The model under review builds one solid part; all positions refer to its coordinate system, in mm. A direction names the side the tool comes from. Coordinates: 2 decimals unless noted, no trailing zeros. Order: outer loops, then holes, each group sorted by start corner. A loop starts at its lowest first (then second) coordinate and runs counter-clockwise, first axis right, second up. Notation, with made-up numbers: M 72,44.25 L 83,44.25 A8 cw 83,57.25 Z; hole C -27.75,80.25 d3. An arc over 180 degrees is marked long. Answer in a Markdown table with one row per item.
Autodesk Inventor part; units mm, degrees
ref_plane "YZ Plane" through (0, 0, 0) normal (1, 0, 0) x (0, 1, 0)
ref_plane "XZ Plane" through (0, 0, 0) normal (0, 1, 0) x (-1, 0, 0)
ref_plane "XY Plane" through (0, 0, 0) normal (0, 0, 1) x (1, 0, 0)
sketch "Sketch1" plane through (0, 0, 0) normal (0, 1, 0) x (-1, 0, 0)
  line L0 (0, 0) -> (47.635, 0)
  line L1 (47.635, 0) -> (47.635, -52.715)
  line L2 (47.635, -52.715) -> (0, -52.715)
  line L3 (0, -52.715) -> (0, 0)
  circle A0 centre (45.725, -1.91) radius 2.1
  circle A1 centre (45.725, -50.805) radius 2.1
  circle A2 centre (1.91, -1.91) radius 2.1
  circle A3 centre (1.91, -50.805) radius 2.1
  line L4 (47.635, 0) -> (51.445, 0)
  line L5 (51.445, 0) -> (51.445, -52.715)
  line L6 (51.445, -52.715) -> (47.635, -52.715)
  line L7 (47.635, -52.715) -> (47.635, 0)
  line L8 (0, 0) -> (-3.81, 0)
  line L9 (-3.81, 0) -> (-3.81, -56.525)
  line L10 (-3.81, -56.525) -> (0, -56.525)
  line L11 (0, -56.525) -> (0, 0)
  line L12 (51.445, -52.715) -> (-6.35, -52.715)
  line L13 (-6.35, -52.715) -> (-6.35, -56.525)
  line L14 (-6.35, -56.525) -> (51.445, -56.525)
  line L15 (51.445, -56.525) -> (51.445, -52.715)
  line L16 (-3.81, 0) -> (51.445, 0)
  line L17 (51.445, 0) -> (51.445, 3.81)
  line L18 (51.445, 3.81) -> (-3.81, 3.81)
  line L19 (-3.81, 3.81) -> (-3.81, 0)
  point P0 (0, -52.715)
  point P1 (0, -51.6779)
  point P2 (0, -49.9321)
  point P3 (0, -2.7829)
  point P4 (0, -1.0371)
  point P5 (-3.81, -77.675)
  point P6 (-3.81, -52.715)
  point P7 (0, -52.715)
  point P8 (1.0371, -52.715)
  point P9 (2.7829, -52.715)
  point P10 (0, -52.715)
  point P11 (0, -56.525)
  point P12 (0, -56.525)
  dimension "d0" = 52.715
  dimension "d1" = 47.635
  dimension "d3" = 4.2
  dimension "d4" = 4.2
  dimension "d6" = 1.91
  dimension "d7" = 1.91
  dimension "d8" = 1.91
  dimension "d9" = 4.2
  dimension "d10" = 4.2
  dimension "d11" = 1.91
  dimension "d12" = 1.91
  dimension "d13" = 1.91
  dimension "d14" = 1.91
  dimension "d15" = 1.91
  dimension "d18" = 3.81
  dimension "d19" = 3.81
  dimension "d20" = 3.81
  dimension "d21" = 3.81
  dimension "d38" = 0
  dimension "d39" = 0
extrude "Extrusion5" add sketch "Sketch1" along normal blind 15 contours L8 L19 L18 L17 L4 L0 A0 A2 | L0 A2 L3 | L3 A2 A3 L12 L9 L8 | L0 A0 L1 A1 L2 A3 L3 A2 | L12 L11 L10 L9 | L3 A3 L2 | L2 A3 A1 L6 L15 L14 L11 | L0 L1 A0 | A0 L1 L4 L5 L6 A1 | L1 L2 A1 picked at (0.2904, -0.2904) picked at (0.2904, -52.4246) picked at (47.3446, -0.2904) picked at (47.3446, -52.4246)
sketch "Sketch6" plane through (0, 15, 0) normal (0, 1, 0) x (1, 0, 0)
  line L0 (-51.445, -3.81) -> (3.81, -3.81)
  line L1 (-51.445, -3.81) -> (-38.745, -3.81)
  line L2 (-38.745, -3.81) -> (-38.745, 8.89)
  line L3 (-38.745, 8.89) -> (-51.445, 8.89)
  line L4 (-51.445, 8.89) -> (-51.445, -3.81)
  line L5 (3.81, 56.525) -> (-51.445, 56.525)
  line L6 (-51.445, 56.525) -> (-38.745, 56.525)
  line L7 (-38.745, 56.525) -> (-38.745, 43.825)
  line L8 (-38.745, 43.825) -> (-51.445, 43.825)
  line L9 (-51.445, 43.825) -> (-51.445, 56.525)
  line L10 (3.81, -3.81) -> (3.81, 56.525)
  line L11 (3.81, 56.525) -> (-8.89, 56.525)
  line L12 (-8.89, 56.525) -> (-8.89, 43.825)
  line L13 (-8.89, 43.825) -> (3.81, 43.825)
  line L14 (3.81, 43.825) -> (3.81, 56.525)
  line L15 (3.81, -3.81) -> (-8.89, -3.81)
  line L16 (-8.89, -3.81) -> (-8.89, 8.89)
  line L17 (-8.89, 8.89) -> (3.81, 8.89)
  line L18 (3.81, 8.89) -> (3.81, -3.81)
  line L19 (3.81, 56.525) -> (-51.445, 56.525)
  line L20 (-51.445, 56.525) -> (-51.445, -3.81)
  line L21 (-51.445, -3.81) -> (3.81, -3.81)
  line L22 (3.81, -3.81) -> (3.81, 56.525)
  circle A0 centre (-1.91, 1.91) radius 2.1
  circle A1 centre (-45.725, 1.91) radius 2.1
  circle A2 centre (-45.725, 50.805) radius 2.1
  circle A3 centre (-1.91, 50.805) radius 2.1
  point P0 (0, 0)
  point P1 (3.81, 8.89)
  dimension "d42" = 12.7
  dimension "d43" = 12.7
  dimension "d44" = 12.7
  dimension "d45" = 12.7
  dimension "d46" = 12.7
  dimension "d47" = 12.7
extrude "Extrusion6" cut sketch "Sketch6" against normal blind 10 contours L2 L3 L20 L8 L7 L5 L12 L13 L10 L17 L16 L0
sketch "Sketch7" plane through (0, 0, 0) normal (0, -1, 0) x (1, 0, 0)
  line L0 (3.81, -56.525) -> (-51.445, -56.525)
  line L1 (3.81, 3.81) -> (3.81, -56.525)
  line L2 (-51.445, 3.81) -> (3.81, 3.81)
  line L3 (-51.445, -56.525) -> (-51.445, 3.81)
  circle A0 centre (-1.91, -1.91) radius 2.1
  circle A1 centre (-45.725, -1.91) radius 2.1
  circle A2 centre (-45.725, -50.805) radius 2.1
  circle A3 centre (-1.91, -50.805) radius 2.1
  line L4 (-8.89, 3.81) -> (3.81, 3.81)
  line L5 (3.81, 3.81) -> (-51.445, 3.81)
  line L6 (-51.445, 3.81) -> (-51.445, 6.35)
  line L7 (-51.445, 6.35) -> (3.81, 6.35)
  line L8 (3.81, 6.35) -> (3.81, 3.81)
  line L9 (-51.445, 6.35) -> (-53.985, 6.35)
  line L10 (-53.985, 6.35) -> (-53.985, -56.525)
  line L11 (-53.985, -56.525) -> (-51.445, -56.525)
  line L12 (-51.445, -56.525) -> (-51.445, 6.35)
  line L13 (-53.985, -56.525) -> (3.81, -56.525)
  line L14 (3.81, -56.525) -> (3.81, -59.065)
  line L15 (3.81, -59.065) -> (-53.985, -59.065)
  line L16 (-53.985, -59.065) -> (-53.985, -56.525)
  line L17 (3.81, -59.065) -> (6.35, -59.065)
  line L18 (6.35, -59.065) -> (6.35, 5.08)
  line L19 (6.35, 5.08) -> (3.81, 5.08)
  line L20 (3.81, 5.08) -> (3.81, -59.065)
  line L21 (6.35, 5.08) -> (3.81, 5.08)
  line L22 (3.81, 5.08) -> (3.81, 6.35)
  line L23 (3.81, 6.35) -> (6.35, 6.35)
  line L24 (6.35, 6.35) -> (6.35, 5.08)
  point P0 (0, 0)
  dimension "d50" = 2.54
  dimension "d51" = 2.54
  dimension "d52" = 2.54
  dimension "d53" = 2.54
extrude "Extrusion7" add sketch "Sketch7" against normal blind 19 contours L14 L15 L16 L11 L0 | L1 L8 L19 L18 L17 L14 | L11 L10 L9 L6 L3 | L2 L6 L7 L8 | L8 L23 L24 L19
sketch "Sketch8" plane through (0, 19, 0) normal (0, 1, 0) x (1, 0, 0)
  line L0 (-53.985, -6.35) -> (6.35, -6.35)
  line L1 (6.35, -6.35) -> (6.35, 59.065)
  line L2 (6.35, 59.065) -> (-53.985, 59.065)
  line L3 (-53.985, 59.065) -> (-53.985, -6.35)
  line L4 (3.81, 56.525) -> (3.81, -3.81)
  line L5 (3.81, -3.81) -> (-51.445, -3.81)
  line L6 (-51.445, -3.81) -> (-51.445, 56.525)
  line L7 (-51.445, 56.525) -> (3.81, 56.525)
  circle A0 centre (-1.91, 50.805) radius 2.1
  line L8 (-1.91, 50.805) -> (-10.17, 50.805)
  line L9 (-10.17, 50.805) -> (-10.17, 48.127)
  line L10 (-10.17, 48.127) -> (-1.91, 48.127)
  line L11 (-1.91, 48.127) -> (-1.91, 50.805)
  line L12 (6.35, 59.065) -> (-53.985, 59.065)
  line L13 (-10.17, 48.127) -> (-22.87, 48.127)
  line L14 (-22.87, 48.127) -> (-22.87, 59.065)
  line L15 (-22.87, 59.065) -> (-10.17, 59.065)
  line L16 (-10.17, 59.065) -> (-10.17, 48.127)
  point P0 (0, 0)
  point P1 (-10.17, 56.525)
  point P2 (-22.87, 56.525)
  dimension "d56" = 8.26
  dimension "d57" = 12.7
extrude "Extrusion8" cut sketch "Sketch8" against normal blind 8 contours L2 L16 L7 L14
sketch "Sketch9" plane through (0, 5, 0) normal (0, 1, 0) x (1, 0, 0)
  point P0 (0, 0)
sketch "Sketch10" plane through (3.81, 19, 3.81) normal (0, 0, -1) x (-1, 0, 0)
  line L0 (36.83, -2.8033) -> (17.78, -2.8033)
  line L1 (17.78, -2.8033) -> (17.78, -11.7199)
  line L2 (17.78, -11.7199) -> (36.83, -11.7199)
  line L3 (36.83, -11.7199) -> (36.83, -2.8033)
  point P0 (3.81, -19)
  point P1 (12.7, -4)
  dimension "d60" = 19.05
  dimension "d61" = 5.08
extrude "Extrusion9" cut sketch "Sketch10" against normal blind 25.4
properties part number "PCB_REMOTE_Holder_tall_"
(1) Take a section at B-B (y = 13.25). Write out the cut boundary in (x, z) (3 decimals).
Report:
| item | result |
|---|---|
| outline | M -53.985,-59.065 L -22.87,-59.065 L -22.87,-56.525 L -38.745,-56.525 L -38.745,-43.825 L -51.445,-43.825 L -51.445,-8.89 L -38.745,-8.89 L -38.745,3.81 L -33.02,3.81 L -33.02,6.35 L -53.985,6.35 Z; M -13.97,3.81 L -8.89,3.81 L -8.89,-8.89 L 3.81,-8.89 L 3.81,-43.825 L -8.89,-43.825 L -8.89,-56.525 L -10.17,-56.525 L -10.17,-59.065 L 6.35,-59.065 L 6.35,6.35 L -13.97,6.35 Z; hole C -45.725,-50.805 d4.2; hole C -45.725,-1.91 d4.2; hole C -1.91,-50.805 d4.2; hole C -1.91,-1.91 d4.2 |
(2) To check wall thickness, follow line 1 (X direction, y = 5.75, z = -1.91) (3 decimals); line 2 (Z direction, x = -1.91, y = 6.75) (3 decimals); line 3 (X direction, y = 15.5, z = -20) (3 decimals). State the ranges of each line that lie inside material, in increasing order. Write a range as [from, to].
Report:
| item | result |
|---|---|
| line 1 | [-53.985, -47.825], [-43.625, -38.745], [-8.89, -4.01], [0.19, 6.35] |
| line 2 | [-59.065, -52.905], [-48.705, -43.825], [-8.89, -4.01], [0.19, 6.35] |
| line 3 | [-53.985, -51.445], [3.81, 6.35] |
(3) Take a section at D-D (x = -12). Write out the cut boundary in (y, z) (3 decimals), then the cut area to 3 significant figures.
Report:
| item | result |
|---|---|
| outline | M 0,-59.065 L 11,-59.065 L 11,-56.525 L 5,-56.525 L 5,3.81 L 19,3.81 L 19,6.35 L 0,6.35 Z |
| area | 378 mm^2 |
(4) Take a section at A-A (z = -1.91). Write out the cut boundary in (x, y) (3 decimals).
Report:
| item | result |
|---|---|
| outline | M -53.985,0 L -47.825,0 L -47.825,15 L -51.445,15 L -51.445,19 L -53.985,19 Z; M -43.625,0 L -4.01,0 L -4.01,15 L -8.89,15 L -8.89,5 L -38.745,5 L -38.745,15 L -43.625,15 Z; M 0.19,0 L 6.35,0 L 6.35,19 L 3.81,19 L 3.81,15 L 0.19,15 Z |
(5) Take a section at C-C (x = -1.91). Write out the cut boundary in (y, z) (3 decimals), then the cut area to 3 significant figures.
Report:
| item | result |
|---|---|
| outline | M 0,-59.065 L 19,-59.065 L 19,-56.525 L 15,-56.525 L 15,-52.905 L 0,-52.905 Z; M 0,-48.705 L 15,-48.705 L 15,-43.825 L 5,-43.825 L 5,-8.89 L 15,-8.89 L 15,-4.01 L 0,-4.01 Z; M 0,0.19 L 15,0.19 L 15,3.81 L 19,3.81 L 19,6.35 L 0,6.35 Z |
| area | 526 mm^2 |
(6) Insertion check: P1, Ø10, axis at x = -46, z = -4, coming from the +Y side; P2, Ø4, axis at x = -1.91, z = -1.91, coming from the +Y side; P3, Ø2, axis at x = -13.5, z = -0.5, coming from the +Y side; P4, Ø2, axis at x = -18, z = -58, coming from the +Y side. Each pin has a flat end and moves straight along its axis. Give the tip position at first contact, or say it passes through.
Report:
| item | result |
|---|---|
| P1 | y = 15 |
| P2 | through |
| P3 | y = 5 |
| P4 | y = 11 |
(7) Machinability: for faces 4 (the cylindrical face through (-43.627, 7.395, -2.002)), 5 (the flat face through (-22.87, 15, -58)), 6 (the flat face through (-8.89, 10, -50)), which of the approach directions +Z, -Z, +X, -X, +Y, -Y give a long, thin tool a straight path to every point of the face, cutting with its end or side? Answer none if there is none.
Report:
| item | result |
|---|---|
| face 4 | +Y, -Y |
| face 5 | -Z, +Y |
| face 6 | +Y |
(8) The part is to be moulded in two halves that separate along Y. For faces 1 (the flat face through (-33.02, 12, 5)), 2 (the flat face through (-1, 15, -48.7)), 3 (the flat face through (-38.745, 10, -50)), say which applies: +Y half, -Y half, draft (parallel to the pull), parting line (faces both ways), or undercut.
Report:
| item | result |
|---|---|
| face 1 | undercut |
| face 2 | +Y half |
| face 3 | draft |
